Read the model definition and answer for the solid it produces. Units are mm, in the model's axes. Face numbers are marked on the shaded views. A direction names the side the tool comes from. Give positions to 0.01 mm unless a question says otherwise; leave off trailing zeros. Loops run counter-clockwise (first coordinate to the right, second up) from the corner with the lowest first, then second, coordinate; pieces in that order, holes last. Notation, with made-up numbers: (63.25, -12.5) - (120.25, -12.5) arc R11 cw to (120.25, 4.5) - close; hole circle Ø5 at (28, -10.75). An arc over 180 degrees is marked (long way). Write item = value, one per line.
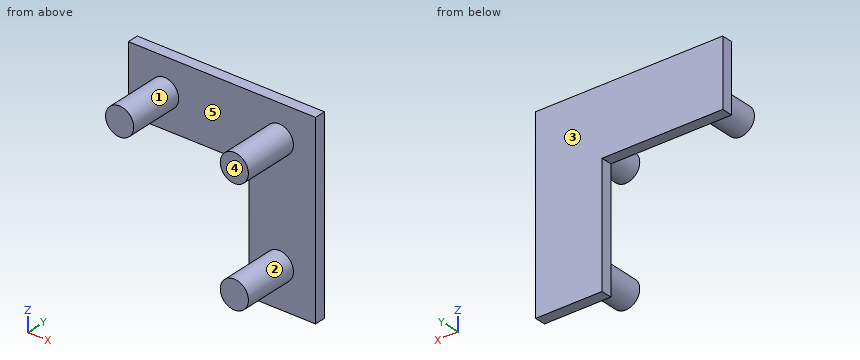
```python
from build123d import *

# Parameters (mm, degrees)
F0_W     = 60
F0_H     = 108.9
F0_R     = 12.7
F1_DEPTH = 10
F2_DEPTH = 60.8


with BuildPart() as f1:
    # F0 (on Front) → F1 (new body)
    with BuildSketch(Plane.XZ):
        with BuildLine():
            Line((-60, 60), (-168.9, 60))
            Line((-168.9, 60), (-168.9, 30))
            Line((-168.9, 30), (-148.9, 30))
            ThreePointArc((-148.9, 30), (-136.2, 42.7), (-123.5, 30))
            Line((-123.5, 30), (-60, 30))
            Line((-60, 30), (-60, 60))
        make_face()
        with BuildLine():
            Line((0, 60), (-60, 60))
            Line((-60, 60), (-60, 30))
            Line((-60, 30), (-45.4, 30))
            ThreePointArc((-45.4, 30), (-32.7, 42.7), (-20, 30))
            Line((-20, 30), (0, 30))
            Line((0, 30), (0, 60))
        make_face()
        with BuildLine():
            Line((-148.9, 30), (-168.9, 30))
            Line((-168.9, 30), (-168.9, 0))
            Line((-168.9, 0), (-60, 0))
            Line((-60, 0), (-60, 30))
            Line((-60, 30), (-123.5, 30))
            ThreePointArc((-123.5, 30), (-136.2, 17.3), (-148.9, 30))
        make_face()
        with BuildLine():
            Line((-45.4, 30), (-60, 30))
            Line((-60, 30), (-60, 0))
            Line((-60, 0), (0, 0))
            Line((0, 0), (0, 30))
            Line((0, 30), (-20, 30))
            ThreePointArc((-20, 30), (-32.7, 17.3), (-45.4, 30))
        make_face()
        with Locations((-30, -54.45)):
            Rectangle(F0_W, F0_H)
        with Locations((-32.7, -73.5)):
            Circle(F0_R, mode=Mode.SUBTRACT)
    extrude(amount=F1_DEPTH)

    # F0 (on Front) → F2 (join)
    with BuildSketch(Plane.XZ):
        with BuildLine():
            Line((-123.5, 30), (-148.9, 30))
            ThreePointArc((-148.9, 30), (-136.2, 17.3), (-123.5, 30))
        make_face()
        with BuildLine():
            ThreePointArc((-123.5, 30), (-136.2, 42.7), (-148.9, 30))
            Line((-148.9, 30), (-123.5, 30))
        make_face()
        with BuildLine():
            ThreePointArc((-20, 30), (-32.7, 42.7), (-45.4, 30))
            Line((-45.4, 30), (-20, 30))
        make_face()
        with BuildLine():
            Line((-20, 30), (-45.4, 30))
            ThreePointArc((-45.4, 30), (-32.7, 17.3), (-20, 30))
        make_face()
        with Locations((-32.7, -73.5)):
            Circle(F0_R)
    extrude(amount=F2_DEPTH)


solid = f1.part
```
1) A cutting plane is placed at C-C on y = -29.5. Determine the outline of the cut face in (x, z), then the cut area to 3 significant figures.
Output:
outline = circle Ø25.4 at (-136.2, 30); circle Ø25.4 at (-32.7, -73.5); circle Ø25.4 at (-32.7, 30)
area = 1,520 mm²
2) A tool of negligible diameter and unlimited length cuts with its end or side. For the marked faces 4 and 5, from which of +Z, -Z, +X, -X, +Y, -Y can it reach the whole face along a straight path? Write none if from no direction.
Output:
face_4 = +Z, -Z, +X, -X, -Y
face_5 = -Y
3) A cutting plane is placed at D-D on z = -73.5. Determine the outline of the cut face in (x, y), then the cut area to 3 significant figures.
Output:
outline = (-60, -10) - (-45.4, -10) - (-45.4, -60.8) - (-20, -60.8) - (-20, -10) - (0, -10) - (0, 0) - (-60, 0) - close
area = 1,890 mm²
4) The mould has two halves that part along X. Classify the marked faces 1, 2 and 3: pulls with the +X half, pulls with the -X half, needs draft (parallel to the pull), parting line crosses it, or undercut.
Output:
face_1 = undercut
face_2 = parting line crosses it
face_3 = needs draft
5) Each of these flat-tipped pins is pushed along its axis until it touches: P1, Ø1, axis at x = -133.5, y = -36.5, coming from the +Z side; P2, Ø6, axis at x = -123.5, z = -4.5, coming from the -Y side; P3, Ø8, axis at x = -110, y = -7.5, coming from the -Z side; P4, Ø2, axis at y = -32.5, z = 21, coming from the +X side. Where does it stop, or does it pass through?
Output:
P1 = 42.51
P2 = through
P3 = 0
P4 = -22.84
6) A cutting plane is placed at B-B on x = -136.2. Determine the outline of the cut face in (y, z), then the cut area to 3 significant figures.
Output:
outline = (-60.8, 17.3) - (-10, 17.3) - (-10, 0) - (0, 0) - (0, 60) - (-10, 60) - (-10, 42.7) - (-60.8, 42.7) - close
area = 1,890 mm²
7) Find the intervals of material crossed by probe 1 along Z at (x, y) = (-119, -4); probe 2 along Z at (x, y) = (-33.5, -38); probe 3 along Z at (x, y) = (-136, -21), in increasing order.
Output:
probe_1 = 0 to 60
probe_2 = -86.17 to -60.83, 17.33 to 42.67
probe_3 = 17.3 to 42.7
8) A cutting plane is placed at A-A on z = 30. Determine the outline of the cut face in (x, y), then the cut area to 3 significant figures.
Output:
outline = (-168.9, -10) - (-148.9, -10) - (-148.9, -60.8) - (-123.5, -60.8) - (-123.5, -10) - (-45.4, -10) - (-45.4, -60.8) - (-20, -60.8) - (-20, -10) - (0, -10) - (0, 0) - (-168.9, 0) - close
area = 4,270 mm²
